Geometry: final body of the model. Coordinates: model frame, mm. A direction names the side the tool comes from. Coordinates: 2 decimals unless noted, no trailing zeros. Loops run counter-clockwise (first coordinate to the right, second up) from the corner with the lowest first, then second, coordinate; pieces in that order, holes last. Notation, with made-up numbers: (84.25, 42) - (127.25, 42) arc R30 cw to (127.25, 76) - close; hole circle Ø6 at (11, 20). An arc over 180 degrees is marked (long way). Put each result on its own line as item: value. Start each with the question number.
1) Section A-A on y = 29. Output: boundary loops of the cut face in (x, z).
2) Section B-B on z = 0. Output: boundary loops of the cut face in (x, y), and give its area (3 significant figures).
3) Draft query along Y for faces 6 (the cylindrical face through (4.38, 271.99, -8.43)), 7 (the flat face through (-2.2, 276.1, 8.4)), 8 (the cylindrical face through (4.57, 277.973, 7.167)), 9 (the flat face through (-0.1, 288, 6.2)). Return one class per face: +Y half, -Y half, draft (parallel to the pull), parting line (faces both ways), or undercut.
4) Contact query for flat-ended pins moving along their axis: pin 1 Ø1 at (y, z) = (45, 3) entering from +X (3 decimals); pin 2 Ø4 at (x, z) = (8.5, -0.5) entering from +Y; pin 3 Ø5 at (x, y) = (-8, 196) entering from -Z. Output: stop coordinate, or through.
5) Material intervals for line 1 along Z through (x, y) = (0, 14); line 2 along Y through (x, z) = (0.5, -2.75); line 3 along Z through (x, y) = (-0.5, 97.5), sorted ascending. Write a range as from..to.
6) Section D-D on y = 291. Output: boundary loops of the cut face in (x, z).
7) Reachability of faces 1 (the cylindrical face through (-12.932, 132.124, 5.362)), 2 (the flat face through (-3, 0, -6)), 3 (the cylindrical face through (-6, 303, 0)), 4 (the flat face through (-2.2, 279.9, 8.4)), 5 (the cylindrical face through (-6, 22, 0)) from +Z, -Z, +X, -X, +Y, -Y: full face, straight path, thin tool, end or side. Return the list, or none.
8) Section C-C on x = 0. Output: boundary loops of the cut face in (y, z), and give its area (3 significant figures).
Autodesk Inventor part; units mm, degrees
ref_plane "YZ Plane" through (0, 0, 0) normal (1, 0, 0) x (0, 1, 0)
ref_plane "XZ Plane" through (0, 0, 0) normal (0, 1, 0) x (-1, 0, 0)
ref_plane "XY Plane" through (0, 0, 0) normal (0, 0, 1) x (1, 0, 0)
sketch "Sketch1" plane through (0, 0, 0) normal (0, 1, 0) x (-1, 0, 0)
  circle A0 centre (0, 0) radius 14
  dimension "d0" = 28
extrude "Extrusion1" add sketch "Sketch1" along normal blind 268
sketch "Sketch5" plane through (0, 268, 0) normal (0, 1, 0) x (1, 0, 0)
  point P0 (0, 0)
sketch "Sketch6" plane through (0, 0, 0) normal (1, 0, 0) x (0, 1, 0)
  point P0 (0, 0)
sketch "Sketch7" plane through (0, 268, 0) normal (0, 1, 0) x (1, 0, 0)
  circle A0 centre (0, 0) radius 9.5
  dimension "d13" = 19
extrude "Extrusion3" add sketch "Sketch7" along normal blind 8.1
sketch "Sketch8" plane through (0, 276.1, 0) normal (0, 1, 0) x (1, 0, 0)
  circle A0 centre (0, 0) radius 8.5
  dimension "d16" = 17
extrude "Extrusion4" add sketch "Sketch8" along normal blind 3.8
sketch "Sketch9" plane through (0, 279.9, 0) normal (0, 1, 0) x (1, 0, 0)
  circle A0 centre (0, 0) radius 9.5
  dimension "d19" = 19
extrude "Extrusion5" add sketch "Sketch9" along normal blind 8.1
sketch "Sketch10" plane through (0, 288, 0) normal (0, 1, 0) x (1, 0, 0)
  circle A0 centre (0, 0) radius 6
  dimension "d22" = 12
extrude "Extrusion6" add sketch "Sketch10" along normal blind 30
sketch "Sketch11" plane through (0, 0, 0) normal (0, -1, 0) x (1, 0, 0)
  circle A0 centre (0, 0) radius 6
  dimension "d25" = 12
extrude "Extrusion7" cut sketch "Sketch11" against normal blind 45
thread "Thread1"
thread "Thread2"
properties part number "Hydraulic cylinder part 3"
Answer block:
1. outline: circle Ø28 at (0, 0); hole circle Ø12 at (0, 0)
2. outline: (-14, 0) - (-6, 0) - (-6, 45) - (6, 45) - (6, 0) - (14, 0) - (14, 268) - (9.5, 268) - (9.5, 276.1) - (8.5, 276.1) - (8.5, 279.9) - (9.5, 279.9) - (9.5, 288) - (6, 288) - (6, 318) - (-6, 318) - (-6, 288) - (-9.5, 288) - (-9.5, 279.9) - (-8.5, 279.9) - (-8.5, 276.1) - (-9.5, 276.1) - (-9.5, 268) - (-14, 268) - close
2. area: 7,700 mm²
3. face 6: draft
3. face 7: undercut
3. face 8: undercut
3. face 9: +Y half
4. pin 1: stops at x = 13.775
4. pin 2: stops at y = 288
4. pin 3: stops at z = -12.87
5. line 1: z = -14..-6, 6..14
5. line 2: y = 45..318
5. line 3: z = -13.99..13.99
6. outline: circle Ø12 at (0, 0)
7. face 1: +Y, -Y
7. face 2: +Z, -Z, +X, -X, -Y
7. face 3: +Y
7. face 4: none
7. face 5: -Y
8. outline: (0, -14) - (268, -14) - (268, -9.5) - (276.1, -9.5) - (276.1, -8.5) - (279.9, -8.5) - (279.9, -9.5) - (288, -9.5) - (288, -6) - (318, -6) - (318, 6) - (288, 6) - (288, 9.5) - (279.9, 9.5) - (279.9, 8.5) - (276.1, 8.5) - (276.1, 9.5) - (268, 9.5) - (268, 14) - (0, 14) - (0, 6) - (45, 6) - (45, -6) - (0, -6) - close
8. area: 7,700 mm²
